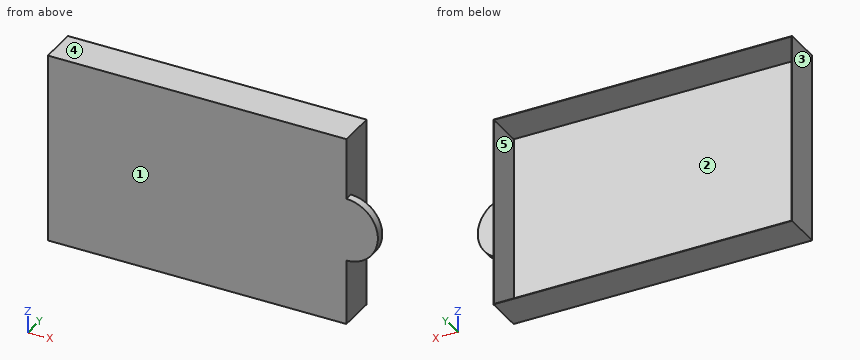
```python
from build123d import *

# Parameters (mm, degrees)
CROQUIS1_W              = 72.404273835
CROQUIS1_H              = 46.251918891
SALIENTE_EXTRUIR1_DEPTH = 9.1
VACIADO2_T              = -0.1
SALIENTE_EXTRUIR2_DEPTH = 2


with BuildPart() as part:
    # Croquis1 → Saliente-Extruir1 (new body)
    with BuildSketch(Plane(origin=(0, 0, 0), x_dir=(1, 0, 0), z_dir=(0, 1, 0))):
        with Locations((36.202136917, 23.125959446)):
            Rectangle(CROQUIS1_W, CROQUIS1_H)
    extrude(amount=SALIENTE_EXTRUIR1_DEPTH)

    # Vaciado2
    vaciado2_openings = [part.faces().sort_by_distance(p)[0] for p in [
        (36.202136917, 9.1, -23.125959446),
    ]]
    offset(amount=VACIADO2_T, openings=vaciado2_openings, kind=Kind.INTERSECTION)

    # Croquis2 → Saliente-Extruir2 (add)
    with BuildSketch(Plane(origin=(0, 0, 0), x_dir=(1, 0, 0), z_dir=(0, 1, 0))):
        with BuildLine():
            Line((72.304273835, 14.936525207), (72.304273835, 30.379638096))
            ThreePointArc((72.304273835, 30.379638096), (80.025830279, 22.658081652), (72.304273835, 14.936525207))
        make_face()
    extrude(amount=SALIENTE_EXTRUIR2_DEPTH)


solid = part.part
```
Could you check a few things on this model? Use its own coordinates, in mm. Face numbers are marked on the shaded views. A direction names the side the tool comes from. Round coordinates to 2 decimals unless told otherwise and drop trailing zeros. Write each loop counter-clockwise with the first axis right and the second up, starting at its lowest first coordinate (ties: lowest second). Pieces come first, ordered by that corner, then holes.
(1) Suppose I cut it at A-A on y = 5.75. Write out the boundary of the cut face in (x, z), and give its area (3 significant figures).
Findings below:
outline: (0, -46.25) - (72.4, -46.25) - (72.4, 0) - (0, 0) - close; hole (0.1, -46.15) - (72.3, -46.15) - (72.3, -0.1) - (0.1, -0.1) - close
area: 23.7 mm2
(2) Suppose I cut it at D-D on y = 1.25. Write out the boundary of the cut face in (x, z), and give its area (3 significant figures).
Findings below:
outline: (0, -46.25) - (72.4, -46.25) - (72.4, -30.38) arc R7.72 ccw to (72.4, -14.94) - (72.4, 0) - (0, 0) - close; hole (0.1, -46.15) - (72.3, -46.15) - (72.3, -0.1) - (0.1, -0.1) - close
area: 116 mm2
(3) Which directions (+Z, -Z, +X, -X, +Y, -Y) give clear straight access to the entire face, cutting with the end or side of a thin tool? Please do the marked faces 1 and 2.
Findings below:
face 1: +Z, -Z, +X, -X, -Y
face 2: +Y
(4) Suppose I cut it at B-B on x = 39. Write out the boundary of the cut face in (y, z), and give its area (3 significant figures).
Findings below:
outline: (0, -46.25) - (9.1, -46.25) - (9.1, -46.15) - (0.1, -46.15) - (0.1, -0.1) - (9.1, -0.1) - (9.1, 0) - (0, 0) - close
area: 6.43 mm2
(5) For pin 1 (3 mm diameter, centred on x = 35.5, z = -11, fed in from +Y); pin 2 (4 mm diameter, centred on x = 70.5, z = -36, fed in from +Y); pin 3 (2.5 mm diameter, centred on y = 4.5, z = -13.5, fed in from +X); pin 4 (2.5 mm diameter, centred on x = 77, z = -21, fed in from +Y), each with a flat end and sliding along its axis, tell me the tip position at first contact or that it passes through.
Findings below:
pin 1: stops at y = 0.1
pin 2: stops at y = 9.1
pin 3: stops at x = 72.4
pin 4: stops at y = 2
(6) If I drill on probe 1 along Y at (x, z) = (75, -29.5), over which ranges is the centre line in solid material (lowest first)?
Findings below:
probe 1: y = 0 to 2
(7) Thinking about a two-plate mould opening in X: for the marked faces 3, 4 and 5, which applies, +X half, -X half, draft (parallel to the pull), parting line (faces both ways), or undercut?
Findings below:
face 3: -X half
face 4: draft
face 5: undercut
(8) Suppose I cut it at C-C on z = -32.5. Write out the boundary of the cut face in (x, y), and give its area (3 significant figures).
Findings below:
outline: (0, 0) - (72.4, 0) - (72.4, 9.1) - (72.3, 9.1) - (72.3, 0.1) - (0.1, 0.1) - (0.1, 9.1) - (0, 9.1) - close
area: 9.04 mm2
